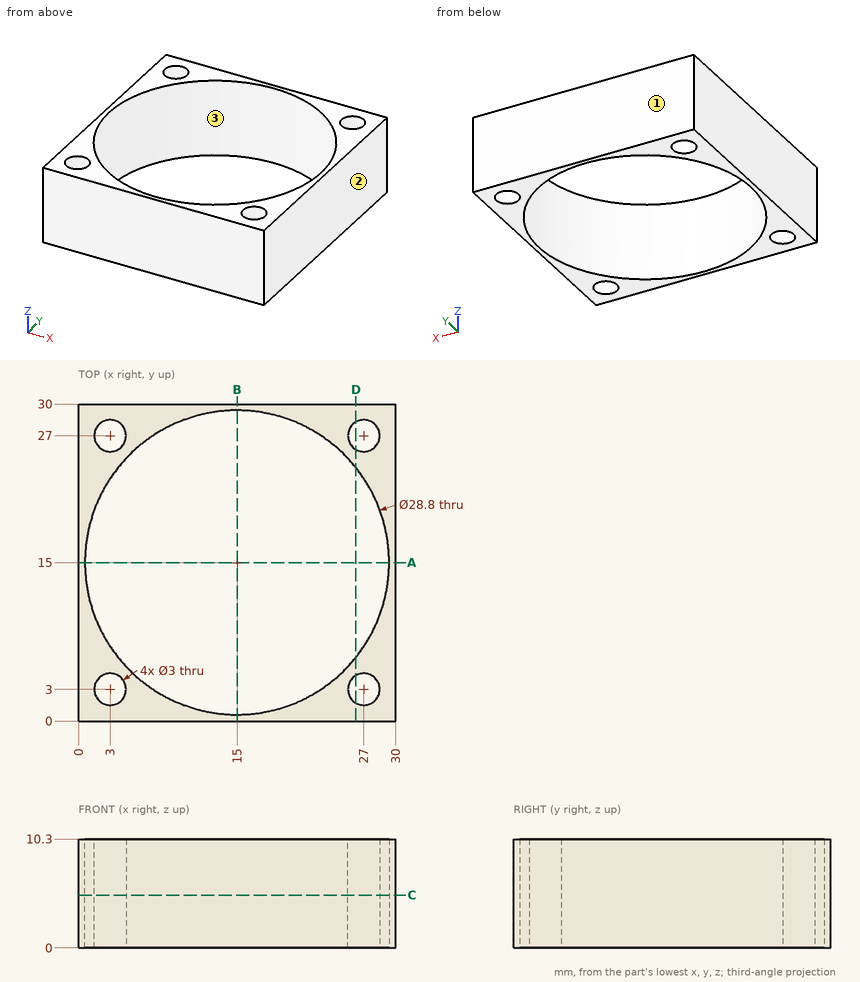
For this review, use the dimensioned drawing (mm, ordinates from the lowest corner) and the shaded views. Coordinates: 2 decimals unless noted, no trailing zeros. Loops run counter-clockwise (first coordinate to the right, second up) from the corner with the lowest first, then second, coordinate; pieces in that order, holes last. Notation, with made-up numbers: (77.5, 45.5) - (96.5, 45.5) arc R17 cw to (96.5, 66.5) - close; hole circle Ø1 at (31.5, 60.25). An arc over 180 degrees is marked (long way). Use one line per item in the form item = value. Start each with the question number.
1) To check wall thickness, follow probe 1 along X at (y, z) = (3, 2.25); probe 2 along X at (y, z) = (23.75, 2.25). State the ranges of each line that lie inside material, in increasing order. Write a range as from..to.
2) Take a section at D-D (x = 26.25). State the section outline as (y, z) points, plus the area to 3 significant figures.
3) Take a section at A-A (y = 15). State the section outline as (x, z) points, plus the area to 3 significant figures.
4) Take a section at C-C (z = 5). State the section outline as (x, y) points.
5) Draft analysis for pull direction X (two halves, no side actions). For the marked faces 1, 2 and 3, state which applies: released by +X, released by -X, zero draft, split by the parting line, or undercut.
From the geometry:
q1.probe_1 = 0..1.5, 4.5..7.04, 22.96..25.5, 28.5..30
q1.probe_2 = 0..3.56, 26.44..30
q2.outline = (0, 0) - (1.7, 0) - (1.7, 10.3) - (0, 10.3) - close; (4.3, 0) - (6.01, 0) - (6.01, 10.3) - (4.3, 10.3) - close; (23.99, 0) - (25.7, 0) - (25.7, 10.3) - (23.99, 10.3) - close; (28.3, 0) - (30, 0) - (30, 10.3) - (28.3, 10.3) - close
q2.area = 70.3 mm2
q3.outline = (0, 0) - (0.6, 0) - (0.6, 10.3) - (0, 10.3) - close; (29.4, 0) - (30, 0) - (30, 10.3) - (29.4, 10.3) - close
q3.area = 12.4 mm2
q4.outline = (0, 0) - (30, 0) - (30, 30) - (0, 30) - close; hole circle Ø28.8 at (15, 15); hole circle Ø3 at (3, 3); hole circle Ø3 at (3, 27); hole circle Ø3 at (27, 3); hole circle Ø3 at (27, 27)
q5.face_1 = zero draft
q5.face_2 = released by +X
q5.face_3 = undercut
